Source: CAD feature listing. Evaluate the final solid. Frame: model axes, mm. A direction names the side the tool comes from. Give positions to 0.01 mm unless a question says otherwise; leave off trailing zeros. Loops run counter-clockwise (first coordinate to the right, second up) from the corner with the lowest first, then second, coordinate; pieces in that order, holes last.
from build123d import *

# Parameters (mm, degrees)
SKETCH_1_W          = 30
SKETCH_1_H          = 30
EXTRUDE_1_DEPTH     = 3
SKETCH_2_R          = 12
EXTRUDE_2_DEPTH     = 1
SKETCH_3_R          = 10
CUT_EXTRUDE_2_DEPTH = 22.587033145
SKETCH_4_R          = 1.6
CUT_EXTRUDE_3_DEPTH = 22.587033145
FILLET_1_R          = 2


with BuildPart() as part:
    # 草图1 → 凸台-拉伸1 (new body)
    with BuildSketch(Plane.XY):
        Rectangle(SKETCH_1_W, SKETCH_1_H)
    extrude(amount=EXTRUDE_1_DEPTH)

    # 草图2 → 凸台-拉伸2 (add)
    with BuildSketch(Plane.XY.offset(3)):
        Circle(SKETCH_2_R)
    extrude(amount=EXTRUDE_2_DEPTH)

    # 草图3 → 切除-拉伸2 (cut, through all)
    with BuildSketch(Plane.XY.offset(4)):
        Circle(SKETCH_3_R)
    extrude(amount=-CUT_EXTRUDE_2_DEPTH, mode=Mode.SUBTRACT)

    # 草图4 → 切除-拉伸3 (cut, through all)
    with BuildSketch(Plane(origin=(0, 0, 0), x_dir=(-1, 0, 0), z_dir=(0, 0, -1))):
        with Locations((12, 12)):
            Circle(SKETCH_4_R)
        with Locations((-12, 12)):
            Circle(SKETCH_4_R)
        with Locations(Location((12, -12, 0), (0, 0, 180))):
            Circle(SKETCH_4_R)
        with Locations(Location((-12, -12, 0), (0, 0, 180))):
            Circle(SKETCH_4_R)
    extrude(amount=-CUT_EXTRUDE_3_DEPTH, mode=Mode.SUBTRACT)

    # 圆角1
    fillet_1_edges = [part.edges().sort_by_distance(p)[0] for p in [
        (-15, 15, 1.5),
        (15, 15, 1.5),
        (15, -15, 1.5),
        (-15, -15, 1.5),
    ]]
    fillet(fillet_1_edges, radius=FILLET_1_R)


solid = part.part
1) Reachability of faces 1 (the flat face through (0, 15, 1)), 2 (the flat face through (-7, 10, 3)) from +Z, -Z, +X, -X, +Y, -Y: full face, straight path, thin tool, end or side. Return the list, or none.
Checks:
face 1: +Z, -Z, +X, -X, +Y
face 2: +Z
2) Cut plane C-C (z = 2.3). Return loops of the section in (x, y), and give its area (3 significant figures).
Checks:
outline: (-15, -13) arc R2 ccw to (-13, -15) - (13, -15) arc R2 ccw to (15, -13) - (15, 13) arc R2 ccw to (13, 15) - (-13, 15) arc R2 ccw to (-15, 13) - close; hole circle Ø3.2 at (-12, -12); hole circle Ø3.2 at (-12, 12); hole circle Ø20 at (0, 0); hole circle Ø3.2 at (12, -12); hole circle Ø3.2 at (12, 12)
area: 550 mm2
3) Pull-direction query (X, two-part tool) for faces 3 (the cylindrical face through (-14.43, 14.4, 1.52)), 4 (the cylindrical face through (-10.4, 12.07, 1.48)), 5 (the cylindrical face through (14.4, 14.43, 1.52)); classes: released by +X, released by -X, zero draft, split by the parting line, or undercut.
Checks:
face 3: released by -X
face 4: undercut
face 5: released by +X
4) Cut plane A-A (x = 0). Return loops of the section in (y, z).
Checks:
outline: (-15, 0) - (-10, 0) - (-10, 4) - (-12, 4) - (-12, 3) - (-15, 3) - close; (10, 0) - (15, 0) - (15, 3) - (12, 3) - (12, 4) - (10, 4) - close
5) Ray query, probe 1 along Y at (x, z) = (-12, 1.8); probe 2 along X at (y, z) = (-13, 1.4). Return the intervals inside material, ascending.
Checks:
probe 1: y = -15 to -13.6, -10.4 to 10.4, 13.6 to 15
probe 2: x = -15 to -13.25, -10.75 to 10.75, 13.25 to 15
6) Cut plane D-D (y = -11.25). Return loops of the section in (x, z).
Checks:
outline: (-15, 0) - (-13.41, 0) - (-13.41, 3) - (-15, 3) - close; (-10.59, 0) - (10.59, 0) - (10.59, 3) - (4.18, 3) - (4.18, 4) - (-4.18, 4) - (-4.18, 3) - (-10.59, 3) - close; (13.41, 0) - (15, 0) - (15, 3) - (13.41, 3) - close
